from build123d import *

# Parameters (mm, degrees)
F1_DEPTH  = 2.54
F2_DEPTH  = 25.4
F3_DEPTH  = 12.7
F4_DEPTH  = 2.54
F6_DEPTH  = 2.54
F7_DEPTH  = 25.4
F9_DEPTH  = 2.54
F10_DEPTH = 25.4


with BuildPart() as f1:
    # F0 (on Top) → F1 (new body)
    with BuildSketch(Plane.XY):
        with BuildLine():
            Line((-19.05, -3.81), (19.05, -3.81))
            ThreePointArc((19.05, -3.81), (15.24, 0), (19.05, 3.81))
            Line((19.05, 3.81), (-19.05, 3.81))
            ThreePointArc((-19.05, 3.81), (-16.355923, 2.694077), (-15.24, 0))
            ThreePointArc((-15.24, 0), (-16.355923, -2.694077), (-19.05, -3.81))
        make_face()
    extrude(amount=F1_DEPTH)

    # F0 (on Top) → F2 (join)
    with BuildSketch(Plane.XY):
        with BuildLine():
            ThreePointArc((19.05, 3.81), (15.24, 0), (19.05, -3.81))
            ThreePointArc((19.05, -3.81), (21.744077, -2.694077), (22.86, 0))
            ThreePointArc((22.86, 0), (21.744077, 2.694077), (19.05, 3.81))
        make_face()
    extrude(amount=F2_DEPTH)

    # F5 (on face) → F6 (join)
    with BuildSketch(Plane.XY.offset(25.4)):
        with BuildLine():
            Line((-19.05, -3.81), (19.05, -3.81))
            ThreePointArc((19.05, -3.81), (22.86, 0), (19.05, 3.81))
            Line((19.05, 3.81), (-19.05, 3.81))
            ThreePointArc((-19.05, 3.81), (-16.355923, 2.694077), (-15.24, 0))
            ThreePointArc((-15.24, 0), (-16.355923, -2.694077), (-19.05, -3.81))
        make_face()
    extrude(amount=F6_DEPTH)

    # F5 (on face) → F7 (join)
    with BuildSketch(Plane.XY.offset(25.4)):
        with BuildLine():
            ThreePointArc((-19.05, 3.81), (-22.86, 0), (-19.05, -3.81))
            ThreePointArc((-19.05, -3.81), (-16.355923, -2.694077), (-15.24, 0))
            ThreePointArc((-15.24, 0), (-16.355923, 2.694077), (-19.05, 3.81))
        make_face()
    extrude(amount=F7_DEPTH)

    # F0 (on Top) → F9 (join)
    with BuildSketch(Plane.XY):
        with BuildLine():
            ThreePointArc((-19.05, 3.81), (-22.86, 0), (-19.05, -3.81))
            ThreePointArc((-19.05, -3.81), (-16.355923, -2.694077), (-15.24, 0))
            ThreePointArc((-15.24, 0), (-16.355923, 2.694077), (-19.05, 3.81))
        make_face()
    extrude(amount=F9_DEPTH)

    # F0 (on Top) → F10 (join)
    with BuildSketch(Plane.XY):
        with BuildLine():
            ThreePointArc((-19.05, 3.81), (-22.86, 0), (-19.05, -3.81))
            ThreePointArc((-19.05, -3.81), (-16.355923, -2.694077), (-15.24, 0))
            ThreePointArc((-15.24, 0), (-16.355923, 2.694077), (-19.05, 3.81))
        make_face()
    extrude(amount=-F10_DEPTH)


with BuildPart() as f3:
    # F0 (on Top) → F3 (new body)
    with BuildSketch(Plane.XY):
        with BuildLine():
            ThreePointArc((-19.05, 3.81), (-22.86, 0), (-19.05, -3.81))
            ThreePointArc((-19.05, -3.81), (-16.355923, -2.694077), (-15.24, 0))
            ThreePointArc((-15.24, 0), (-16.355923, 2.694077), (-19.05, 3.81))
        make_face()
    extrude(amount=-F3_DEPTH)


with BuildPart() as f4:
    # F0 (on Top) → F4 (new body)
    with BuildSketch(Plane.XY):
        with BuildLine():
            ThreePointArc((-19.05, 3.81), (-22.86, 0), (-19.05, -3.81))
            ThreePointArc((-19.05, -3.81), (-16.355923, -2.694077), (-15.24, 0))
            ThreePointArc((-15.24, 0), (-16.355923, 2.694077), (-19.05, 3.81))
        make_face()
    extrude(amount=F4_DEPTH)


solid = f1.part
Geometry check sheet. Reference: the model listing, model coordinates, mm. Round coordinates to 2 decimals unless told otherwise and drop trailing zeros. Order: outer loops, then holes, each group sorted by start corner. A loop starts at its lowest first (then second) coordinate and runs counter-clockwise, first axis right, second up. Notation, with made-up numbers: M -12.5,14.5 L 25.5,14.5 A13 ccw 25.5,24.5 Z; hole C 40.25,7 d1. An arc over 180 degrees is marked long. Answer in a Markdown table with one row per item. Add a question column.
Item 1: Sectioned sample at A-A, the plane x = 10.5. Enter the section's corners in (y, z), plus the area to 3 significant figures.
Item 2: Sectioned sample at C-C, the plane z = 15. Enter the section's corners in (x, y).
Item 3: Draft check along Z on faces 1 (the face through (-19, 0, -25.4)), 2 (the face through (-2, 0, 2.54)), 3 (the face through (-19, 0, 50.8)), 4 (the face through (0, -3.81, 1)). Enter one of: released by +Z, released by -Z, zero draft, split by the parting line, or undercut.
Item 4: Material ranges on L1, parallel to Z at x = -4.5, y = 3.5; L2, parallel to Z at x = -16, y = 1; L3, parallel to Z at x = 20.5, y = -2.5, recorded low to high. Write a range as [from, to].
Item 5: Depth check by flat-ended pin: pin 1 Ø2.5 at (x, y) = (-11.5, -1.5) entering from -Z; pin 2 Ø2 at (x, y) = (0, -2.5) entering from +Z. Enter the tip coordinate at first touch or a pass-through.
Item 6: Sectioned sample at B-B, the plane y = 1.75. Enter the section's corners in (x, z), plus the area to 3 significant figures.
Filled in:
| question | item | result |
|---|---|---|
| 1 | outline | M -3.81,0 L 3.81,0 L 3.81,2.54 L -3.81,2.54 Z; M -3.81,25.4 L 3.81,25.4 L 3.81,27.94 L -3.81,27.94 Z |
| 1 | area | 38.7 mm² |
| 2 | outline | M 19.05,-3.81 A3.81 ccw 22.86,0 A3.81 ccw long Z |
| 3 | face 1 | released by -Z |
| 3 | face 2 | undercut |
| 3 | face 3 | released by +Z |
| 3 | face 4 | zero draft |
| 4 | L1 | z = [0, 2.54], [25.4, 27.94] |
| 4 | L2 | z = [-25.4, 2.54], [25.4, 50.8] |
| 4 | L3 | z = [0, 27.94] |
| 5 | pin 1 | stops at z = 0 |
| 5 | pin 2 | stops at z = 27.94 |
| 6 | outline | M -22.43,-25.4 L -15.67,-25.4 L -15.67,0 L 22.43,0 L 22.43,27.94 L -15.67,27.94 L -15.67,50.8 L -22.43,50.8 L -22.43,25.4 L 15.67,25.4 L 15.67,2.54 L -22.43,2.54 Z |
| 6 | area | 709 mm² |
